For this review, use the dimensioned drawing (mm, ordinates from the lowest corner) and the shaded views. A direction names the side the tool comes from. Round coordinates to 2 decimals unless told otherwise and drop trailing zeros. Loops run counter-clockwise (first coordinate to the right, second up) from the corner with the lowest first, then second, coordinate; pieces in that order, holes last. Notation, with made-up numbers: M 44.25,81 L 63.25,81 A26 ccw 63.25,120 Z; hole C 43.5,32.5 d4. An arc over 180 degrees is marked long. One line per item, written item: value. Start each with the question number.
Item 1: We need section A-A (z = 19). Write out the cut boundary in (x, y), then the cut area to 3 significant figures.
Item 2: We need section C-C (y = 2.75). Write out the cut boundary in (x, z), then the cut area to 3 significant figures.
Item 3: For the marked faces 5 and 6, list the 3-axis set-ups (+Z, -Z, +X, -X, +Y, -Y) from which the entire face can be reached by the end or side of a thin tool; tool diameter is ignored.
Item 4: Mouldability with a two-part tool opening along X and no side actions: class the marked faces 1, 2, 3 and 4 as released by +X, released by -X, zero draft, split by the parting line, or undercut.
Item 5: We need section D-D (z = 5). Write out the cut boundary in (x, y).
Item 6: We need section B-B (x = 9.25). Write out the cut boundary in (y, z), then the cut area to 3 significant figures.
Item 7: For line 1 along X through (y, z) = (1.9, 19); line 2 along Z through (x, y) = (10, 0.5); line 3 along X through (y, z) = (0.7, 5), list the stretches that pass through material, from the lowest coordinate up.
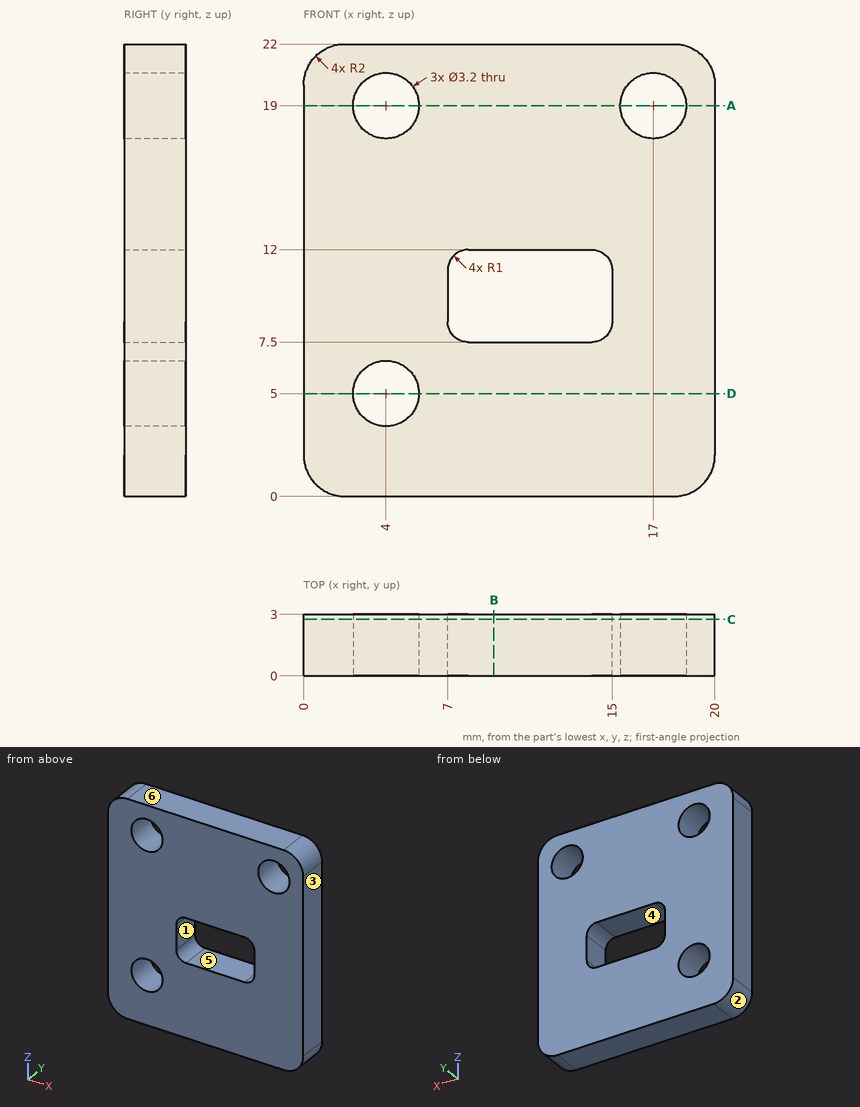
A:
1. outline: M 0,0 L 2.4,0 L 2.4,3 L 0,3 Z; M 5.6,0 L 15.4,0 L 15.4,3 L 5.6,3 Z; M 18.6,0 L 20,0 L 20,3 L 18.6,3 Z
1. area: 40.8 mm2
2. outline: M 0,2 A2 ccw 2,0 L 18,0 A2 ccw 20,2 L 20,20 A2 ccw 18,22 L 2,22 A2 ccw 0,20 Z; hole C 4,5 d3.2; hole C 4,19 d3.2; hole M 7,8.5 A1 ccw 8,7.5 L 14,7.5 A1 ccw 15,8.5 L 15,11 A1 ccw 14,12 L 8,12 A1 ccw 7,11 Z; hole C 17,19 d3.2
2. area: 377 mm2
3. face 5: +Y, -Y
3. face 6: +Z, +X, -X, +Y, -Y
4. face 1: undercut
4. face 2: released by -X
4. face 3: released by +X
4. face 4: undercut
5. outline: M 0,0 L 2.4,0 L 2.4,3 L 0,3 Z; M 5.6,0 L 20,0 L 20,3 L 5.6,3 Z
6. outline: M 0,0 L 3,0 L 3,7.5 L 0,7.5 Z; M 0,12 L 3,12 L 3,22 L 0,22 Z
6. area: 52.5 mm2
7. line 1: 0 to 2.4, 5.6 to 15.4, 18.6 to 20
7. line 2: 0 to 7.5, 12 to 22
7. line 3: 0 to 2.4, 5.6 to 20
